from build123d import *

# Parameters (mm, degrees)
BOSS_EXTRUDE1_DEPTH         = 6.35
FILLET1_R                   = 3
CUT_EXTRUDE1_REACH          = 82.301
TAP_DRILL_FOR_M5X0_8_TAP1_D = 4.2


with BuildPart() as part:
    # Sketch1 → Boss-Extrude1 (new body)
    with BuildSketch(Plane.XY):
        with BuildLine():
            Line((18, 0), (18, -78))
            Line((18, -78), (-18, -78))
            Line((-18, -78), (-18, 0))
            ThreePointArc((-18, 0), (0, -18), (18, 0))
        make_face()
    extrude(amount=BOSS_EXTRUDE1_DEPTH)

    # Fillet1
    fillet1_edges = [part.edges().sort_by_distance(p)[0] for p in [
        (18, 0, 3.175),
        (18, -78, 3.175),
        (-18, -78, 3.175),
        (-18, 0, 3.175),
    ]]
    fillet(fillet1_edges, radius=FILLET1_R)

    # Sketch2 → Cut-Extrude1 (cut, up to next)
    with BuildSketch(Plane.XY.offset(6.35), mode=Mode.PRIVATE) as cut_extrude1_sk1:
        with BuildLine():
            Line((-12.61, -72), (-12.61, -64))
            ThreePointArc((-12.61, -64), (-10, -61.39), (-7.39, -64))
            Line((-7.39, -64), (-7.39, -72))
            ThreePointArc((-7.39, -72), (-10, -74.61), (-12.61, -72))
        make_face()
    cut_extrude1_tool1 = extrude(cut_extrude1_sk1.sketch, amount=-CUT_EXTRUDE1_REACH, mode=Mode.PRIVATE) & part.part
    # Sketch2 → Cut-Extrude1 (cut, up to next)
    with BuildSketch(Plane.XY.offset(6.35), mode=Mode.PRIVATE) as cut_extrude1_sk2:
        with BuildLine():
            Line((-12.61, -52), (-12.61, -44))
            ThreePointArc((-12.61, -44), (-10, -41.39), (-7.39, -44))
            Line((-7.39, -44), (-7.39, -52))
            ThreePointArc((-7.39, -52), (-10, -54.61), (-12.61, -52))
        make_face()
    cut_extrude1_tool2 = extrude(cut_extrude1_sk2.sketch, amount=-CUT_EXTRUDE1_REACH, mode=Mode.PRIVATE) & part.part
    # Sketch2 → Cut-Extrude1 (cut, up to next)
    with BuildSketch(Plane.XY.offset(6.35), mode=Mode.PRIVATE) as cut_extrude1_sk3:
        with BuildLine():
            Line((12.61, -72), (12.61, -64))
            ThreePointArc((12.61, -64), (10, -61.39), (7.39, -64))
            Line((7.39, -64), (7.39, -72))
            ThreePointArc((7.39, -72), (10, -74.61), (12.61, -72))
        make_face()
    cut_extrude1_tool3 = extrude(cut_extrude1_sk3.sketch, amount=-CUT_EXTRUDE1_REACH, mode=Mode.PRIVATE) & part.part
    # Sketch2 → Cut-Extrude1 (cut, up to next)
    with BuildSketch(Plane.XY.offset(6.35), mode=Mode.PRIVATE) as cut_extrude1_sk4:
        with BuildLine():
            Line((12.61, -52), (12.61, -44))
            ThreePointArc((12.61, -44), (10, -41.39), (7.39, -44))
            Line((7.39, -44), (7.39, -52))
            ThreePointArc((7.39, -52), (10, -54.61), (12.61, -52))
        make_face()
    cut_extrude1_tool4 = extrude(cut_extrude1_sk4.sketch, amount=-CUT_EXTRUDE1_REACH, mode=Mode.PRIVATE) & part.part
    add(cut_extrude1_tool1.solids().sort_by_distance((-10, -68, 6.35))[0], mode=Mode.SUBTRACT)
    add(cut_extrude1_tool2.solids().sort_by_distance((-10, -48, 6.35))[0], mode=Mode.SUBTRACT)
    add(cut_extrude1_tool3.solids().sort_by_distance((10, -68, 6.35))[0], mode=Mode.SUBTRACT)
    add(cut_extrude1_tool4.solids().sort_by_distance((10, -48, 6.35))[0], mode=Mode.SUBTRACT)

    # Tap Drill for M5x0.8 Tap1 (through all)
    with Locations(Plane(origin=(-10, -22.912878475, 6.35), x_dir=(1, 0, 0), z_dir=(0, 0, 1))):
        with Locations((0, 0), (20, 0)):
            Hole(TAP_DRILL_FOR_M5X0_8_TAP1_D / 2)


solid = part.part
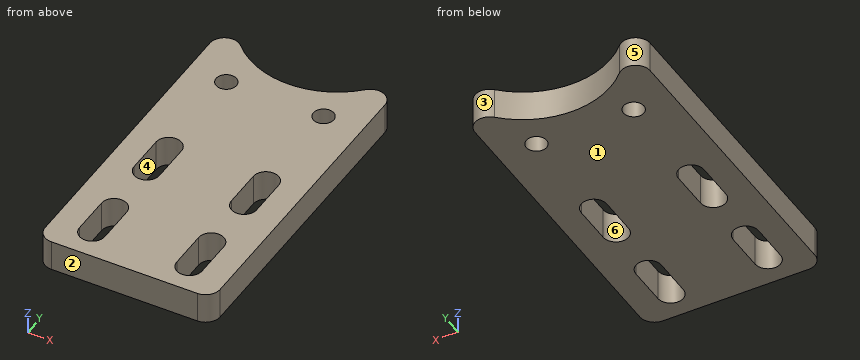
CAD build for the part. Positions are in the model's coordinates, mm. Face numbers are marked on the shaded views. A direction names the side the tool comes from. Round coordinates to 2 decimals unless told otherwise and drop trailing zeros. Order: outer loops, then holes, each group sorted by start corner. A loop starts at its lowest first (then second) coordinate and runs counter-clockwise, first axis right, second up. Notation, with made-up numbers: M -17,87.5 L 33,87.5 A22 ccw 33,102.5 Z; hole C 17,58.5 d10. An arc over 180 degrees is marked long. Use one line per item in the form item = value.
Q1. Flat gauge pins, fed straight in: P1, Ø1.5, axis at x = 0.5, z = 4, coming from the +Y side; P2, Ø3.5, axis at x = -10, y = -22.91, coming from the +Z side. Where does each tip first touch, or does it go through?
Recorded:
P1 = -17.96
P2 = through
Q2. Probe L1, parallel to X at y = -48.5, z = 5.25; L2, parallel to Y at x = -10, z = 2; L3, parallel to X at y = -74, z = 1.25. List the from-to ranges inside material, lowest first.
Recorded:
L1 = -18 to -12.61, -7.39 to 7.39, 12.61 to 18
L2 = -78 to -74.61, -61.39 to -54.61, -41.39 to -25.01, -20.81 to -14.97
L3 = -18 to -11.68, -8.32 to 8.32, 11.68 to 18
Q3. Which spindle directions (+Z, -Z, +X, -X, +Y, -Y) get a long thin tool onto all of the face, cutting with end or side? Do the marked faces 5 and 6. Say none if no direction does.
Recorded:
face_5 = +Z, -Z, +Y
face_6 = +Z, -Z
Q4. Saw through at D-D on x = -4.5. Give the cut face in (y, z).
Recorded:
outline = M -78,0 L -17.43,0 L -17.43,6.35 L -78,6.35 Z
Q5. Saw through at A-A on y = -66.5. Give the cut face in (x, z).
Recorded:
outline = M -18,0 L -12.61,0 L -12.61,6.35 L -18,6.35 Z; M -7.39,0 L 7.39,0 L 7.39,6.35 L -7.39,6.35 Z; M 12.61,0 L 18,0 L 18,6.35 L 12.61,6.35 Z
Q6. Saw through at C-C on z = 3.5. Give the cut face in (x, y), then the cut area to 3 significant figures.
Recorded:
outline = M -18,-75 A3 ccw -15,-78 L 15,-78 A3 ccw 18,-75 L 18,-14.7 A3 ccw 12.86,-12.6 A18 cw -12.86,-12.6 A3 ccw -18,-14.7 Z; hole M -12.61,-72 A2.61 ccw -7.39,-72 L -7.39,-64 A2.61 ccw -12.61,-64 Z; hole M -12.61,-52 A2.61 ccw -7.39,-52 L -7.39,-44 A2.61 ccw -12.61,-44 Z; hole C -10,-22.91 d4.2; hole M 7.39,-72 A2.61 ccw 12.61,-72 L 12.61,-64 A2.61 ccw 7.39,-64 Z; hole M 7.39,-52 A2.61 ccw 12.61,-52 L 12.61,-44 A2.61 ccw 7.39,-44 Z; hole C 10,-22.91 d4.2
area = 1,980 mm^2
Q7. Two-plate mould, pull along Y, no slides. Class the marked faces 1, 2, 3 and 4: +Y half, -Y half, draft (parallel to the pull), parting line (faces both ways), or undercut.
Recorded:
face_1 = draft
face_2 = -Y half
face_3 = +Y half
face_4 = undercut
Q8. Saw through at B-B on x = -10. Give the cut face in (y, z), then the cut area to 3 significant figures.
Recorded:
outline = M -78,0 L -74.61,0 L -74.61,6.35 L -78,6.35 Z; M -61.39,0 L -54.61,0 L -54.61,6.35 L -61.39,6.35 Z; M -41.39,0 L -25.01,0 L -25.01,6.35 L -41.39,6.35 Z; M -20.81,0 L -14.97,0 L -14.97,6.35 L -20.81,6.35 Z
area = 206 mm^2
